Design review of the part built by this model. Coordinates are the model's own, in mm. A direction names the side the tool comes from. Give positions to 0.01 mm unless a question says otherwise; leave off trailing zeros. Loops run counter-clockwise (first coordinate to the right, second up) from the corner with the lowest first, then second, coordinate; pieces in that order, holes last. Notation, with made-up numbers: (42.25, 4) - (86.25, 4) arc R18 cw to (86.25, 24) - close; hole circle Ø6 at (50, 3). An arc over 180 degrees is marked (long way). Put each result on its own line as item: value. Start each with the question number.
```python
from build123d import *

# Parameters (mm, degrees)
SKETCH1_W           = 240
SKETCH1_H           = 40
BOSS_EXTRUDE1_DEPTH = 10
SKETCH2_W           = 20
SKETCH2_H           = 40
BOSS_EXTRUDE2_DEPTH = 240
SKETCH3_R           = 2.6
CUT_EXTRUDE1_DEPTH  = 300
SKETCH4_W           = 10
SKETCH4_H           = 40
SKETCH4_W_2         = 180
CUT_EXTRUDE2_DEPTH  = 300
SKETCH5_R           = 2.125
CUT_EXTRUDE3_DEPTH  = 300


with BuildPart() as part:
    # Sketch1 → Boss-Extrude1 (new body)
    with BuildSketch(Plane.XY):
        with Locations((120, 20)):
            Rectangle(SKETCH1_W, SKETCH1_H)
    extrude(amount=BOSS_EXTRUDE1_DEPTH)

    # Sketch2 → Boss-Extrude2 (add)
    with BuildSketch(Plane(origin=(240, 0, 0), x_dir=(0, 0, -1), z_dir=(1, 0, 0))):
        with Locations((-20, 20)):
            Rectangle(SKETCH2_W, SKETCH2_H)
        with BuildLine():
            Line((-30, 40), (-30, 0))
            ThreePointArc((-30, 0), (-50, 20), (-30, 40))
        make_face()
    extrude(amount=-BOSS_EXTRUDE2_DEPTH)

    # Sketch3 → Cut-Extrude1 (cut)
    with BuildSketch(Plane(origin=(240, 0, 0), x_dir=(0, 0, -1), z_dir=(1, 0, 0))):
        with Locations((-35, 20)):
            Circle(SKETCH3_R)
    extrude(amount=-CUT_EXTRUDE1_DEPTH, mode=Mode.SUBTRACT)

    # Sketch4 → Cut-Extrude2 (cut)
    with BuildSketch(Plane.XZ):
        with Locations((15, 30)):
            Rectangle(SKETCH4_W, SKETCH4_H)
        with Locations((120, 30)):
            Rectangle(SKETCH4_W_2, SKETCH4_H)
        with Locations((225, 30)):
            Rectangle(SKETCH4_W, SKETCH4_H)
    extrude(amount=-CUT_EXTRUDE2_DEPTH, mode=Mode.SUBTRACT)

    # Sketch5 → Cut-Extrude3 (cut)
    with BuildSketch(Plane(origin=(0, 0, 0), x_dir=(-1, 0, 0), z_dir=(0, 0, -1))):
        with Locations((-180, 20)):
            Circle(SKETCH5_R)
        with Locations((-120, 20)):
            Circle(SKETCH5_R)
        with Locations((-60, 20)):
            Circle(SKETCH5_R)
    extrude(amount=-CUT_EXTRUDE3_DEPTH, mode=Mode.SUBTRACT)


solid = part.part
```
Item 1: For L1, parallel to X at y = 13.5, z = 10.5; L2, parallel to Y at x = 60, z = 2.5 (3 decimals); L3, parallel to Z at x = 195, y = 15.5, list the stretches that pass through material, from the lowest coordinate up. Write a range as from..to.
Item 2: Consider section C-C (y = 20). Count the separate pieces of the cut face and the enclosed holes in it, plus the area to 3 significant figures.
Item 3: For P1, Ø6, axis at y = 20, z = 35, coming from the +X side; P2, Ø7, axis at x = 60, y = 20, coming from the +Z side; P3, Ø8, axis at x = 12.5, y = 26.5, coming from the +Z side, all flat-tipped, find the tip position at first contact; note any pin that passes through.
Item 4: Consider section A-A (z = 42). State the section outline as (x, y) points.
Item 5: Machinability: for faces 4 (the flat face through (10, 20, 30)), 5 (the cylindrical face through (5.07, 22.578, 35.338)), which of the approach directions +Z, -Z, +X, -X, +Y, -Y give a long, thin tool a straight path to every point of the face, cutting with its end or side? Answer none if there is none.
Item 6: Mouldability with a two-part tool opening along X and no side actions: class faces 1 (the cylindrical face through (25, 20, 50)), 2 (the cylindrical face through (62.123, 20.093, 4.93)), 3 (the flat face through (0, 20, 25)) as pulls with the +X half, pulls with the -X half, needs draft (parallel to the pull), parting line crosses it, or undercut.
Item 7: Consider section D-D (x = 27.5). State the section outline as (y, z) points, plus the area to 3 significant figures.
Item 8: Consider section B-B (x = 120). State the section outline as (y, z) points (3 decimals), plus the area to 4 significant figures.
Geometry says:
1. L1: x = 0..10, 20..30, 210..220, 230..240
1. L2: y = 0..17.875, 22.125..40
1. L3: z = 0..10
2. separate pieces: 8
2. enclosed holes: 0
2. area: 3,660 mm2
3. P1: stops at x = 240
3. P2: stops at z = 10
3. P3: stops at z = 49.71
4. outline: (0, 4) - (10, 4) - (10, 36) - (0, 36) - close; (20, 4) - (30, 4) - (30, 36) - (20, 36) - close; (210, 4) - (220, 4) - (220, 36) - (210, 36) - close; (230, 4) - (240, 4) - (240, 36) - (230, 36) - close
5. face 4: +Z, +Y, -Y
5. face 5: +X, -X
6. face 1: needs draft
6. face 2: undercut
6. face 3: pulls with the -X half
7. outline: (0, 0) - (40, 0) - (40, 30) arc R20 ccw to (0, 30) - close; hole circle Ø5.2 at (20, 35)
7. area: 1,810 mm2
8. outline: (0, 0) - (17.875, 0) - (17.875, 10) - (0, 10) - close; (22.125, 0) - (40, 0) - (40, 10) - (22.125, 10) - close
8. area: 357.5 mm2
